Geometry check sheet. Reference: the model listing, model coordinates, mm. Face numbers are marked on the shaded views. A direction names the side the tool comes from. Coordinates: 2 decimals unless noted, no trailing zeros. Write each loop counter-clockwise with the first axis right and the second up, starting at its lowest first coordinate (ties: lowest second). Pieces come first, ordered by that corner, then holes. Notation, with made-up numbers: M 76.25,73 L 83.25,73 A20 ccw 83.25,106 Z; hole C 17,59.5 d11. An arc over 180 degrees is marked long. Put each result on its own line as item: value. Start each with the question number.
1) Mould release check, pull along Z, two halves, no side actions. Record for the marked faces 1 and 2: released by +Z, released by -Z, zero draft, split by the parting line, or undercut.
2) Cross-section at B-B on z = -47.5. Record the cut outline in (x, y), plus the area to 3 significant figures.
3) Gauge pin test, flat ends, axial feed: pin 1 (3 mm diameter, centred on y = -2, z = 50.5, fed in from +X); pin 2 (1 mm diameter, centred on y = -1.5, z = 39.5, fed in from -X); pin 3 (2.5 mm diameter, centred on x = 51, y = -3, fed in from -Z); pin 4 (2.5 mm diameter, centred on x = -15, z = -18.25, fed in from +Y). Record the tip position at first contact, or that the pin passes through.
4) Cross-section at A-A on x = -15. Record the cut outline in (y, z).
5) Scan lines: line 1 along Z through (x, y) = (-5, -3); line 2 along Z through (x, y) = (-15, -3.55); line 3 along Z through (x, y) = (-26.5, -3.5). Record each from-to range of solid material in increasing order.
6) Cross-section at C-C on z = 40.5. Record the cut outline in (x, y), plus the area to 3 significant figures.
7) Cross-section at D-D on x = 14. Record the cut outline in (y, z).
8) Set-up check for the marked faces 3 and 4: record each of +Z, -Z, +X, -X, +Y, -Y from which the full face is reachable in a straight line by a thin tool's end or side.
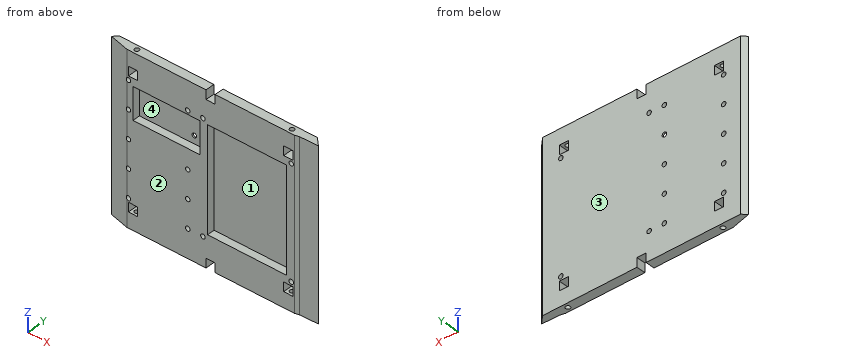
from build123d import *

# Parameters (mm, degrees)
F0_W      = 140
F0_H      = 110
F1_DEPTH  = 6
F3_D      = 3
F3_DEPTH  = 10
F3_TIP    = 0.9012909285
F5_D      = 3
F5_DEPTH  = 10
F5_TIP    = 0.9012909285
F6_SIZE   = 5
F7_W      = 6
F7_H      = 6
F8_DEPTH  = 6.001
F9_W      = 52
F9_H      = 68
F9_W_2    = 44
F9_H_2    = 21
F10_DEPTH = 5
F11_R     = 1.5
F12_DEPTH = 25
F14_DEPTH = 110.001
F16_DEPTH = 110.001


with BuildPart() as f1:
    # F0 (on Front) → F1 (new body)
    with BuildSketch(Plane.XZ):
        Rectangle(F0_W, F0_H)
    extrude(amount=F1_DEPTH)

    # F3
    with Locations(Plane(origin=(0, 0, -55), x_dir=(1, 0, 0), z_dir=(0, 0, -1))):
        with Locations((-51, 3), (51, 3)):
            Hole(F3_D / 2, depth=F3_DEPTH)
            with Locations((0, 0, -(F3_DEPTH + F3_TIP / 2))):  # 118° drill point
                Cone(0, F3_D / 2, F3_TIP, mode=Mode.SUBTRACT)

    # F5
    with Locations(Plane.XY.offset(55)):
        with Locations((51, -3), (-51, -3)):
            Hole(F5_D / 2, depth=F5_DEPTH)
            with Locations((0, 0, -(F5_DEPTH + F5_TIP / 2))):  # 118° drill point
                Cone(0, F5_D / 2, F5_TIP, mode=Mode.SUBTRACT)

    # F6
    f6_edges = [f1.edges().sort_by_distance(p)[0] for p in [
        (-70, 0, 0),
        (70, 0, 0),
    ]]
    chamfer(f6_edges, length=F6_SIZE)

    # F7 (on face) → F8 (cut, through all)
    with BuildSketch(Plane.XZ.offset(6)):
        with Locations((-51, -42)):
            Rectangle(F7_W, F7_H)
        with Locations((51, -42)):
            Rectangle(F7_W, F7_H)
        with Locations((51, 42)):
            Rectangle(F7_W, F7_H)
        with Locations((-51, 42)):
            Rectangle(F7_W, F7_H)
        with Locations((0, -52)):
            Rectangle(F7_W, F7_H)
        with Locations((0, 52)):
            Rectangle(F7_W, F7_H)
    extrude(amount=-F8_DEPTH, mode=Mode.SUBTRACT)

    # F9 (on face) → F10 (cut)
    with BuildSketch(Plane.XZ.offset(6)):
        with Locations((24, 0)):
            Rectangle(F9_W, F9_H)
        with Locations((-29, 23.5)):
            Rectangle(F9_W_2, F9_H_2)
    extrude(amount=-F10_DEPTH, mode=Mode.SUBTRACT)

    # F11 (on face) → F12 (cut)
    with BuildSketch(Plane.XZ.offset(6)):
        with Locations((-54, 36.5)):
            Circle(F11_R)
        with Locations((-5, 36.5)):
            Circle(F11_R)
        with Locations((-15, 36.5)):
            Circle(F11_R)
        with Locations((53, 36.5)):
            Circle(F11_R)
        with Locations((-54, 18.25)):
            Circle(F11_R)
        with Locations((-15, 18.25)):
            Circle(F11_R)
        with Locations((-54, 0)):
            Circle(F11_R)
        with Locations((-15, 0)):
            Circle(F11_R)
        with Locations((-54, -36.5)):
            Circle(F11_R)
        with Locations((-5, -36.5)):
            Circle(F11_R)
        with Locations((-15, -36.5)):
            Circle(F11_R)
        with Locations((53, -36.5)):
            Circle(F11_R)
        with Locations((-54, -18.25)):
            Circle(F11_R)
        with Locations((-15, -18.25)):
            Circle(F11_R)
    extrude(amount=-F12_DEPTH, mode=Mode.SUBTRACT)

    # F13 (on face) → F14 (cut, through all)
    with BuildSketch(Plane(origin=(0, 0, -55), x_dir=(1, 0, 0), z_dir=(0, 0, -1))):
        Polygon((70, 6), (55.0561677185, 6), (57.8561677185, 5.3), (69.95113754, 4.95113754), (70, 5), align=None)
    extrude(amount=-F14_DEPTH, mode=Mode.SUBTRACT)

    # F15 (on face) → F16 (cut, through all)
    with BuildSketch(Plane(origin=(0, 0, -55), x_dir=(1, 0, 0), z_dir=(0, 0, -1))):
        Polygon((-70, 5), (-67.8, 2.8), (-55, 6), (-70, 6), align=None)
    extrude(amount=-F16_DEPTH, mode=Mode.SUBTRACT)


solid = f1.part
Answer key:
1. face 1: undercut
1. face 2: zero draft
2. outline: M -67.8,-2.8 L -55,-6 L 55.06,-6 L 57.86,-5.3 L 69.95,-4.95 L 65,0 L -65,0 Z; hole C -51,-3 d3; hole C 51,-3 d3
2. area: 764 mm²
3. pin 1: stops at x = 68.5
3. pin 2: stops at x = -67
3. pin 3: stops at z = -39
3. pin 4: passes through
4. outline: M -6,-55 L 0,-55 L 0,-38 L -6,-38 Z; M -6,-35 L 0,-35 L 0,-19.75 L -6,-19.75 Z; M -6,-16.75 L 0,-16.75 L 0,-1.5 L -6,-1.5 Z; M -6,1.5 L 0,1.5 L 0,16.75 L -1,16.75 L -1,13 L -6,13 Z; M -6,34 L -1,34 L -1,19.75 L 0,19.75 L 0,35 L -6,35 Z; M -6,38 L 0,38 L 0,55 L -6,55 Z
5. line 1: z = -55 to -38, -35 to 35, 38 to 55
5. line 2: z = -55 to -38, -35 to -19.75, -16.75 to -1.5, 1.5 to 13, 34 to 35, 38 to 55
5. line 3: z = -55 to 13, 34 to 55
6. outline: M -67.8,-2.8 L -55,-6 L -54,-6 L -54,0 L -65,0 Z; M -48,-6 L 48,-6 L 48,0 L -48,0 Z; M 54,-6 L 55.06,-6 L 57.86,-5.3 L 69.95,-4.95 L 65,0 L 54,0 Z
6. area: 706 mm²
7. outline: M -6,-55 L 0,-55 L 0,55 L -6,55 L -6,34 L -1,34 L -1,-34 L -6,-34 Z
8. face 3: +Z, -Z, +X, -X, +Y
8. face 4: -Y
